Autodesk Inventor part; units mm, degrees
ref_plane "YZ Plane" through (0, 0, 0) normal (1, 0, 0) x (0, 1, 0)
ref_plane "XZ Plane" through (0, 0, 0) normal (0, 1, 0) x (-1, 0, 0)
ref_plane "XY Plane" through (0, 0, 0) normal (0, 0, 1) x (1, 0, 0)
sketch "スケッチ1" plane through (0, 0, 0) normal (0, 0, 1) x (1, 0, 0)
  circle A0 centre (211.0538, -16.1783) radius 3
  circle A1 centre (195.0769, -15.1842) radius 3
  circle A2 centre (213.5911, -31.9837) radius 3
  line L0 (195.0769, -15.1842) -> (213.5911, -31.9837) construction
  line L1 (185.1065, 0.6143) -> (518.3624, -301.7771) construction
  circle A3 centre (185.1065, 0.6143) radius 8
  line L2 (204.334, -23.584) -> (211.0538, -16.1783) construction
  line L3 (185.1065, 0.6143) -> (181.7466, -3.0885)
  line L4 (181.7466, -3.0885) -> (195.0769, -15.1842)
  line L5 (211.0538, -16.1783) -> (195.0769, -15.1842) construction
  line L6 (213.748, -11.3362) -> (182.759, -9.4081)
  line L7 (186.8707, -14.4897) -> (289.472, -107.5885)
  arc A4 (195.3874, -10.1938) -> (196.9446, -10.5462) centre (195.0769, -15.1842) ccw
  arc A5 (214.4137, -12.4754) -> (211.3643, -11.1879) centre (211.0538, -16.1783) ccw
  line L8 (214.4137, -12.4754) -> (302.9116, -92.7771)
  line L9 (302.9116, -92.7771) -> (289.472, -107.5885) construction
  circle A6 centre (295.8489, -93.1201) radius 3.025
  circle A7 centre (285.4262, -97.1659) radius 3.025
  circle A8 centre (283.9998, -82.3684) radius 3.025
  line L10 (281.7596, -80.3356) -> (285.1195, -76.6328)
  line L11 (285.1195, -76.6328) -> (289.5999, -80.6983)
  line L12 (289.5999, -80.6983) -> (286.24, -84.4011)
  line L13 (286.24, -84.4011) -> (281.7596, -80.3356) construction
  arc A9 (282.4058, -101.1768) -> (291.3448, -101.5663) centre (287.1097, -95.9928) ccw
  line L14 (302.9116, -92.7771) -> (291.3448, -101.5663)
  arc A10 (299.0788, -95.6895) -> (299.3467, -89.5424) centre (296.6588, -92.5047) ccw
  circle A11 centre (295.8489, -93.1201) radius 1.5
  circle A12 centre (285.4262, -97.1659) radius 1.5
  line L15 (213.5911, -31.9837) -> (181.7466, -3.0885) construction
  line L16 (215.607, -29.762) -> (183.7626, -0.8668)
  line L17 (179.7307, -5.3102) -> (211.5751, -34.2054)
  arc A13 (211.5751, -34.2054) -> (215.607, -29.762) centre (213.5911, -31.9837) ccw
  arc A14 (183.7626, -0.8668) -> (179.7307, -5.3102) centre (181.7466, -3.0885) ccw
  line L18 (211.0538, -16.1783) -> (189.2132, 3.6395) construction
  line L19 (209.0378, -18.4) -> (187.1973, 1.4178)
  line L20 (191.2292, 5.8612) -> (213.0697, -13.9566)
  arc A15 (209.0378, -18.4) -> (213.0697, -13.9566) centre (211.0538, -16.1783) ccw
  arc A16 (191.2292, 5.8612) -> (187.1973, 1.4178) centre (189.2132, 3.6395) ccw
  circle A17 centre (195.0769, -15.1842) radius 1.5
  circle A18 centre (211.0538, -16.1783) radius 1.5
  circle A19 centre (213.5911, -31.9837) radius 1.5
  circle A20 centre (283.9998, -82.3684) radius 1.5
  circle A21 centre (233.2708, -36.3377) radius 3.025
  circle A22 centre (235.8081, -52.1431) radius 3.025
  circle A23 centre (259.1907, -59.857) radius 3.025
  circle A24 centre (261.728, -75.6625) radius 3.025
  line L21 (211.0538, -16.1783) -> (283.9998, -82.3684) construction
  line L22 (285.4262, -97.1659) -> (213.5911, -31.9837) construction
  circle A25 centre (233.2708, -36.3377) radius 1.5
  circle A26 centre (235.8081, -52.1431) radius 1.5
  circle A27 centre (259.1907, -59.857) radius 1.5
  circle A28 centre (261.728, -75.6625) radius 1.5
  point P0 (0, 0)
  point P1 (0, 0)
  point P2 (207.6939, -19.8811)
  point P3 (191.717, -18.887)
  point P4 (197.6688, -17.5361)
  point P5 (200.1335, -6.2694)
  point P6 (209.9194, -11.098)
  point P7 (200.3333, -10.5016)
  point P8 (194.1305, -10.2746)
  point P9 (196.0232, -20.0938)
  point P10 (289.5999, -80.6983)
  point P11 (286.24, -84.4011)
  point P12 (190.0986, -14.718)
  dimension "d13" = 6.05
  dimension "d0" = 6
  dimension "d1" = 25
  dimension "d2" = 10
  dimension "d3" = 18
  dimension "d4" = 5
  dimension "d5" = 5
  dimension "d6" = 150
  dimension "d7" = 6.05
  dimension "d8" = 5
  dimension "d9" = 5
  dimension "d10" = 6.05
  dimension "d11" = 5
  dimension "d12" = 10
  dimension "d14" = 5
  dimension "d15" = 16
  dimension "d16" = 4
  dimension "d17" = 7
  dimension "d18" = 4
  dimension "d19" = 3
  dimension "d20" = 3
  dimension "d23" = 3
  dimension "d24" = 3
  dimension "d25" = 3
  dimension "d26" = 3
  dimension "d29" = 30
  dimension "d30" = 30
  dimension "d31" = 35
  dimension "d32" = 35
  dimension "d33" = 3
  dimension "d34" = 3
  dimension "d35" = 3
  dimension "d36" = 3
extrude "押し出し1" add sketch "スケッチ1" along normal blind 5 contours A0 L20 L6 A5 L8 L10 A8 L12 A10 L14 A9 L7 A4 L17 A2 L16 L19 | L8 L12 A8 L10 | A8 | L17 A4 | A6 | A7
extrude "押し出し2" add sketch "スケッチ1" along normal blind 4 contours A0 | A0 L19 L6 L20 | L16 A1 L4 A4 | L4 A1 L17 A4 | L16 A4 L17 A1 | A1 | L16 A2 L17 A4 | A2 | A21 | A22 | A23 | A24
properties part number "アーム先1" material "ポリカーボネート、スモーク"
The listing builds one solid part. Answer for the finished solid, in the listing's coordinates (mm). A direction names the side the tool comes from. Coordinates: 2 decimals unless noted, no trailing zeros. Loops run counter-clockwise (first coordinate to the right, second up) from the corner with the lowest first, then second, coordinate; pieces in that order, holes last. Notation, with made-up numbers: M 21.5,52.5 L 31.5,52.5 A20 ccw 31.5,83.5 Z; hole C 24,70 d11. An arc over 180 degrees is marked long. Answer as CSV lines item,"result". Start each with the question number.
(1) The part is cut by section C-C (y = -69). Give the vertices of the cut face in (x, z), and give its area (3 significant figures).
(2) For faces 5 (the flat face through (204.75, -14.51, 4.49)), 6 (the cylindrical face through (286.23, -98.43, 2.46)), 7 (the flat face through (211.472, -12.507, 4.493)), determine the directions among +Z, -Z, +X, -X, +Y, -Y from which every point of the face is accessible in a straight line to the end or side of a thin tool.
(3) Find the intervals of material crossed by L1, parallel to Y at x = 295, z = 1.7; L2, parallel to Y at x = 196, z = 1.7; L3, parallel to X at y = -75.5, z = 1, in increasing order. Write a range as [from, to].
(4) The mould has two halves that part along Y. Classify faces 1 (the flat face through (203.5, -10.7, 2.5)), 2 (the cylindrical face through (212.44, -15.6, 1.97)), 3 (the cylindrical face through (294.35, -93.19, 2.46)), 4 (the flat face through (249, -56, 5)): pulls with the +Y half, pulls with the -Y half, needs draft (parallel to the pull), parting line crosses it, or undercut.
(5) The part is cut by section A-A (z = 2.95). State how many separate pieces and enclosed holes the cut face has, and give its area (3 significant figures).
(6) The part is cut by section B-B (x = 271). Give the vertices of the cut face in (y, z).
(7) Given pin 1 (1.8 mm diameter, centred on x = 237, y = -52, fed in from +Z); pin 2 (1 mm diameter, centred on y = -20.5, z = 3.5, fed in from +X); pin 3 (1.8 mm diameter, centred on x = 259.19, y = -59.86, fed in from +Z); pin 4 (2 mm diameter, centred on y = -92, z = 4, fed in from -X), each flat-ended and moving along its own axis, determine where each tip first touches the part or whether it passes through.
Determined:
1,outline,"M 246.94,0 L 276.71,0 L 276.71,5 L 246.94,5 Z"
1,area,"149 mm2"
2,face 5,"+Z, +Y"
2,face 6,"+Z, -Z"
2,face 7,"+Z"
3,L1,"[-98.79, -94.36], [-91.88, -85.6]"
3,L2,"[-22.77, -16.37], [-14, -10.23]"
3,L3,"[254.11, 260.24], [263.22, 283.87]"
4,face 1,"pulls with the +Y half"
4,face 2,"undercut"
4,face 3,"undercut"
4,face 4,"needs draft"
5,separate pieces,"1"
5,enclosed holes,"10"
5,area,"2,510 mm2"
6,outline,"M -90.83,0 L -63.82,0 L -63.82,5 L -90.83,5 Z"
7,pin 1,"z = 4"
7,pin 2,"x = 223.81"
7,pin 3,"through"
7,pin 4,"x = 271.19"
